from build123d import *

# Parameters (mm, degrees)
SKIZZE1_R                            = 25
SKIZZE1_R_2                          = 18.5
AUFSATZ_LINEAR_AUSTRAGEN1_DEPTH      = 18.5
SKIZZE2_R                            = 18.5
SKIZZE2_R_2                          = 15
AUFSATZ_LINEAR_AUSTRAGEN2_DEPTH      = 11.3
SKIZZE3_R                            = 21.5
AUFSATZ_LINEAR_AUSTRAGEN3_DEPTH      = 16
SKIZZE4_R                            = 1.95
SCHNITT_LINEAR_AUSTRAGEN1_DEPTH      = 4.2
SKIZZE5_OUTSIDE_W                    = 64.09
SKIZZE5_OUTSIDE_H                    = 71.09
SKIZZE5_OUTSIDE_W_2                  = 37
SKIZZE5_OUTSIDE_H_2                  = 50
SCHNITT_LINEAR_AUSTRAGEN2_DEPTH      = 35.5000001
SCHNITT_LINEAR_AUSTRAGEN2_DEPTH_BACK = 35.5000001


with BuildPart() as part:
    # Skizze1 → Aufsatz-Linear austragen1 (new body, symmetric)
    with BuildSketch(Plane(origin=(0, 0, 0), x_dir=(1, 0, 0), z_dir=(0, 1, 0))):
        Circle(SKIZZE1_R)
        Circle(SKIZZE1_R_2, mode=Mode.SUBTRACT)
    extrude(amount=AUFSATZ_LINEAR_AUSTRAGEN1_DEPTH, both=True)

    # Skizze2 → Aufsatz-Linear austragen2 (add, symmetric)
    with BuildSketch(Plane(origin=(0, 0, 0), x_dir=(1, 0, 0), z_dir=(0, 1, 0))):
        Circle(SKIZZE2_R)
        Circle(SKIZZE2_R_2, mode=Mode.SUBTRACT)
    extrude(amount=AUFSATZ_LINEAR_AUSTRAGEN2_DEPTH, both=True)

    # Skizze3 → Aufsatz-Linear austragen3 (add)
    with BuildSketch(Plane(origin=(18.5, 0, 0), x_dir=(0, 0, -1), z_dir=(1, 0, 0))):
        Circle(SKIZZE3_R)
    aufsatz_linear_austragen3 = extrude(amount=AUFSATZ_LINEAR_AUSTRAGEN3_DEPTH)

    # Skizze4 → Schnitt-Linear austragen1 (cut)
    with BuildSketch(Plane(origin=(34.5, 0, 0), x_dir=(0, 0, -1), z_dir=(1, 0, 0))):
        with Locations((-5.5, 0)):
            Circle(SKIZZE4_R)
        with Locations((0, 5.5)):
            Circle(SKIZZE4_R)
        with Locations((5.5, 0)):
            Circle(SKIZZE4_R)
        with Locations((0, -5.5)):
            Circle(SKIZZE4_R)
    schnitt_linear_austragen1 = extrude(amount=-SCHNITT_LINEAR_AUSTRAGEN1_DEPTH, mode=Mode.SUBTRACT)

    # Spiegeln1: Aufsatz-Linear austragen3, Schnitt-Linear austragen1 across plane
    add(aufsatz_linear_austragen3.mirror(Plane(origin=(0, 0, 0), x_dir=(0, 0, 1), z_dir=(1, 0, 0))))
    add(schnitt_linear_austragen1.mirror(Plane(origin=(0, 0, 0), x_dir=(0, 0, 1), z_dir=(1, 0, 0))), mode=Mode.SUBTRACT)

    # Skizze5 outside → Schnitt-Linear austragen2 (cut, two sides)
    with BuildSketch(Plane(origin=(0, 29.28598322, 0), x_dir=(0, -1, 0), z_dir=(-1, 0, 0))) as schnitt_linear_austragen2_sk:
        with Locations((29.286, 0)):
            Rectangle(SKIZZE5_OUTSIDE_W, SKIZZE5_OUTSIDE_H)
        with Locations((29.28598322, 0)):
            Rectangle(SKIZZE5_OUTSIDE_W_2, SKIZZE5_OUTSIDE_H_2, mode=Mode.SUBTRACT)
    extrude(amount=SCHNITT_LINEAR_AUSTRAGEN2_DEPTH, mode=Mode.SUBTRACT)
    extrude(schnitt_linear_austragen2_sk.sketch, amount=-SCHNITT_LINEAR_AUSTRAGEN2_DEPTH_BACK, mode=Mode.SUBTRACT)


solid = part.part
Geometry: final body of the model. Coordinates: model frame, mm. A direction names the side the tool comes from. Give positions to 0.01 mm unless a question says otherwise; leave off trailing zeros. Loops run counter-clockwise (first coordinate to the right, second up) from the corner with the lowest first, then second, coordinate; pieces in that order, holes last. Notation, with made-up numbers: (61.5, 86.5) -> (82.5, 86.5) arc R22 ccw to (82.5, 114.5) -> close; hole circle Ø7 at (-30.5, 10). An arc over 180 degrees is marked (long way). Put each result on its own line as item: value.
1. Cut plane C-C (x = 0). Return the cut outline in (y, z), plus the area to 3 significant figures.
Taken from the geometry:
outline: (-18.5, -25) -> (18.5, -25) -> (18.5, -18.5) -> (11.3, -18.5) -> (11.3, -15) -> (-11.3, -15) -> (-11.3, -18.5) -> (-18.5, -18.5) -> close; (-18.5, 18.5) -> (-11.3, 18.5) -> (-11.3, 15) -> (11.3, 15) -> (11.3, 18.5) -> (18.5, 18.5) -> (18.5, 25) -> (-18.5, 25) -> close
area: 639 mm2
2. Set-up query: faces 1 (the cylindrical face through (-4.01, 14.85, 18.06)), 2 (the flat face through (30.3, -5, 0)), 3 (the cylindrical face through (26.388, 0.312, 21.498)), 4 (the cylindrical face through (-32.429, 0.086, -3.552)), 5 (the cylindrical face through (-4.01, -14.95, 18.06)). Return all of +Z, -Z, +X, -X, +Y, -Y with unobstructed straight access to the full face (end or side cutting, diameter ignored); none if empty.
Taken from the geometry:
face 1: +Y
face 2: +X
face 3: +Z, +X
face 4: -X
face 5: -Y
3. Pin query (flat end, axial travel): P1, Ø1.5, axis at x = 8, z = 11.5, coming from the +Y side; P2, Ø6, axis at y = 5.5, z = 0, coming from the +X side; P3, Ø1.2, axis at y = 6, z = -1, coming from the +X side; P4, Ø8, axis at x = 11.5, z = 5.5, coming from the +Y side. Return the tip coordinate at first contact, or that it passes through.
Taken from the geometry:
P1: passes through
P2: stops at x = 34.5
P3: stops at x = 30.3
P4: stops at y = 11.3
4. Cut plane D-D (z = 9.5). Return the cut outline in (x, y), plus the area to 3 significant figures.
Taken from the geometry:
outline: (-34.5, -18.5) -> (-15.87, -18.5) -> (-15.87, -11.3) -> (-11.61, -11.3) -> (-11.61, 11.3) -> (-15.87, 11.3) -> (-15.87, 18.5) -> (-34.5, 18.5) -> close; (11.61, -11.3) -> (15.87, -11.3) -> (15.87, -18.5) -> (34.5, -18.5) -> (34.5, 18.5) -> (15.87, 18.5) -> (15.87, 11.3) -> (11.61, 11.3) -> close
area: 1,570 mm2
5. Ray query, line 1 along Y through (x, z) = (-33, 0); line 2 along Y through (x, z) = (-33, -5.5); line 3 along X through (y, z) = (4.5, 0). Return the intervals inside material, ascending. Write a range as [from, to].
Taken from the geometry:
line 1: y = [-18.5, -7.45], [-3.55, 3.55], [7.45, 18.5]
line 2: y = [-18.5, -1.95], [1.95, 18.5]
line 3: x = [-30.3, -15], [15, 30.3]
6. Pull-direction query (X, two-part tool) for faces 6 (the cylindrical face through (32.429, -7.404, 0.423)), 7 (the cylindrical face through (0, 0, 25)), 8 (the flat face through (30.3, 0, 6)); classes: released by +X, released by -X, zero draft, split by the parting line, or undercut.
Taken from the geometry:
face 6: zero draft
face 7: undercut
face 8: released by +X
